Could you check a few things on this drawing? It's one solid part, dimensions in mm from its lowest x, y, z. A direction names the side the tool comes from. Give positions to 0.01 mm unless a question says otherwise; leave off trailing zeros. Order: outer loops, then holes, each group sorted by start corner. A loop starts at its lowest first (then second) coordinate and runs counter-clockwise, first axis right, second up.
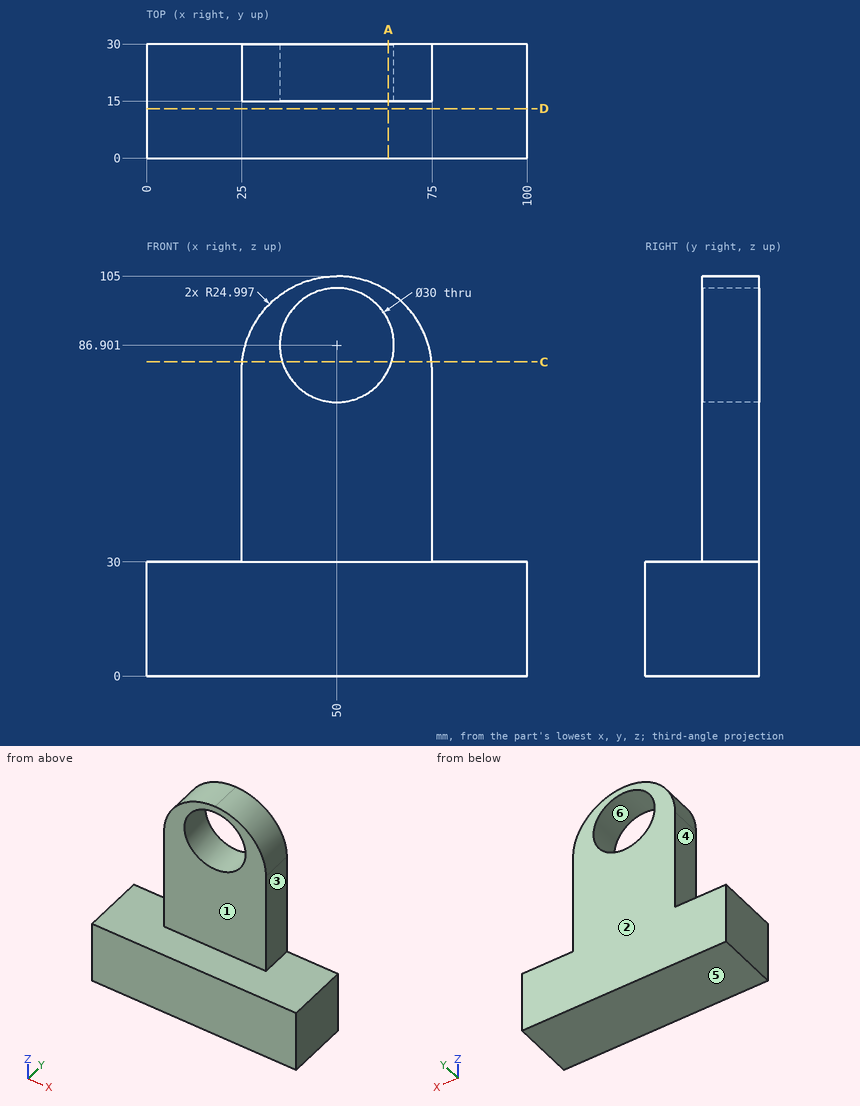
Q1. For the marked faces 1, 2 and 3, which set-ups out of +Z, -Z, +X, -X, +Y, -Y let a thin tool reach every point of the face, with its end or its side?
Filled sheet:
face 1: +Z, +X, -X, -Y
face 2: +Z, -Z, +X, -X, +Y
face 3: +Z, +X, +Y, -Y
Q2. If we section it at A-A on x = 63.5: List the corners of the cut face in (y, z) for me, plus the area to 3 significant figures.
Filled sheet:
outline: (0, 0) - (30, 0) - (30, 80.36) - (15, 80.36) - (15, 30) - (0, 30) - close; (15, 93.44) - (30, 93.44) - (30, 101.04) - (15, 101.04) - close
area: 1,770 mm2
Q3. I need wall thicknesses on L1, parallel to Z at x = 50, y = 18.25; L2, parallel to Y at x = 30, z = 66; L3, parallel to Z at x = 54, y = 23.5 (1 decimal). Which ranges of each line are inside material? Lowest first, please.
Filled sheet:
L1: z = 0 to 71.9, 101.9 to 105
L2: y = 15 to 30
L3: z = 0 to 72.4, 101.4 to 104.7
Q4. If we section it at C-C on z = 82.5: List the corners of the cut face in (x, y) for me (1 decimal), plus the area to 3 significant figures.
Filled sheet:
outline: (25.1, 15) - (35.7, 15) - (35.7, 30) - (25.1, 30) - close; (64.3, 15) - (74.9, 15) - (74.9, 30) - (64.3, 30) - close
area: 316 mm2
Q5. If we section it at D-D on y = 13: List the corners of the cut face in (x, z) for me, plus the area to 3 significant figures.
Filled sheet:
outline: (0, 0) - (100, 0) - (100, 30) - (0, 30) - close
area: 3,000 mm2
Q6. Thinking about a two-plate mould opening in X: for the marked faces 4, 5 and 6, which applies, released by +X, released by -X, zero draft, split by the parting line, or undercut?
Filled sheet:
face 4: released by -X
face 5: zero draft
face 6: undercut
Q7. I'm going to push flat-ended pins straight in: P1, Ø4.5, axis at y = 19, z = 60.5, coming from the +X side; P2, Ø4, axis at y = 21, z = 56, coming from the -X side; P3, Ø15, axis at x = 42.5, z = 83.5, coming from the -Y side. Where does each tip first touch, or does it pass through?
Filled sheet:
P1: stops at x = 75
P2: stops at x = 25
P3: stops at y = 15
